from build123d import *

# Parameters (mm, degrees)
SKETCH7_R           = 2.5
BOSS_EXTRUDE3_DEPTH = 37
SKETCH8_W           = 15.4
SKETCH8_H           = 31
SKETCH8_W_2         = 8.010366446
SKETCH8_W_3         = 36.155804789
CUT_EXTRUDE4_DEPTH  = 76.893008599


with BuildPart() as part:
    # Sketch7 → Boss-Extrude3 (new body)
    with BuildSketch(Plane(origin=(0, 0, 0), x_dir=(1, 0, 0), z_dir=(0, 1, 0))):
        with BuildLine():
            Line((13.729937465, 55.269451431), (59.029937465, 55.269451431))
            ThreePointArc((59.029937465, 55.269451431), (65.129937465, 49.169451431), (59.029937465, 43.069451431))
            Line((59.029937465, 43.069451431), (13.729937465, 43.069451431))
            ThreePointArc((13.729937465, 43.069451431), (7.629937465, 49.169451431), (13.729937465, 55.269451431))
        make_face()
        with Locations(Location((13.729937465, 49.169451431, 0), (0, 0, 270))):
            Circle(SKETCH7_R, mode=Mode.SUBTRACT)
        with Locations(Location((59.029937465, 49.169451431, 0), (0, 0, 270))):
            Circle(SKETCH7_R, mode=Mode.SUBTRACT)
    extrude(amount=BOSS_EXTRUDE3_DEPTH)

    # Sketch8 → Cut-Extrude4 (cut, through all)
    with BuildSketch(Plane(origin=(0, 0, -55.269451431), x_dir=(-1, 0, 0), z_dir=(0, 0, -1))):
        with Locations((-21.429937465, 18.5)):
            Rectangle(SKETCH8_W, SKETCH8_H)
        with Locations((-9.724754242, 18.5)):
            Rectangle(SKETCH8_W_2, SKETCH8_H)
        with Locations((-50.207839859, 18.5)):
            Rectangle(SKETCH8_W_3, SKETCH8_H)
    extrude(amount=-CUT_EXTRUDE4_DEPTH, mode=Mode.SUBTRACT)


solid = part.part
The listing builds one solid part. Answer for the finished solid, in the listing's coordinates (mm). A direction names the side the tool comes from. Round coordinates to 2 decimals unless told otherwise and drop trailing zeros. Loops run counter-clockwise (first coordinate to the right, second up) from the corner with the lowest first, then second, coordinate; pieces in that order, holes last. Notation, with made-up numbers: M 86.25,52.5 L 115.25,52.5 A27 cw 115.25,68.5 Z; hole C -25,-30 d10. An arc over 180 degrees is marked long. Return JSON: item names as keys, results as strings.
Q1. Find section A-A, the plane x = 37. Determine the outline of the cut face in (y, z).
Results list:
{"outline": "M 0,-55.27 L 3,-55.27 L 3,-43.07 L 0,-43.07 Z; M 34,-55.27 L 37,-55.27 L 37,-43.07 L 34,-43.07 Z"}
Q2. The mould has two halves that part along Y. Classify faces 1 (the face through (37, 37, -49)), 2 (the face through (7.63, 1.48, -49.04)), 3 (the face through (29.13, 18, -49)), 4 (the face through (49, 34, -49)): released by +Y, released by -Y, zero draft, split by the parting line, or undercut.
Results list:
{"face 1": "released by +Y", "face 2": "zero draft", "face 3": "undercut", "face 4": "undercut"}
Q3. Find section C-C, the plane z = -52.5. Determine the outline of the cut face in (x, y), plus the area to 3 significant figures.
Results list:
{"outline": "M 8.62,0 L 64.14,0 L 64.14,3 L 32.13,3 L 32.13,34 L 64.14,34 L 64.14,37 L 8.62,37 L 8.62,34 L 29.13,34 L 29.13,3 L 8.62,3 Z", "area": "426 mm2"}
Q4. Each of these flat-tipped pins is pushed along its axis until it touches: pin 1 Ø5 at (y, z) = (29.5, -52) entering from +X; pin 2 Ø1 at (y, z) = (30, -50) entering from -X. Where does it stop, or does it pass through?
Results list:
{"pin 1": "stops at x = 32.13", "pin 2": "stops at x = 29.13"}
Q5. Which of the six approach directions +Z, -Z, +X, -X, +Y, -Y give full straight-line access (tool end or side, diameter ignored) to faces 5 (the face through (32.13, 18, -49)), 6 (the face through (18, 34, -49)), 7 (the face through (31, 20, -55.269))?
Results list:
{"face 5": "+Z, -Z, +X", "face 6": "+Z, -Z, -X", "face 7": "-Z, +X, -X, +Y, -Y"}
Q6. Find the intervals of material crossed by line 1 along Y through (x, z) = (50.5, -47.25); line 2 along X through (y, z) = (15, -45.25); line 3 along X through (y, z) = (2, -53.75), in increasing order. Write a range as from..to.
Results list:
{"line 1": "y = 0..3, 34..37", "line 2": "x = 29.13..32.13", "line 3": "x = 9.7..63.06"}
Q7. Find section D-D, the plane x = 58. Determine the outline of the cut face in (y, z), plus the area to 3 significant figures.
Results list:
{"outline": "M 0,-55.27 L 3,-55.27 L 3,-51.45 L 0,-51.45 Z; M 0,-46.89 L 3,-46.89 L 3,-43.07 L 0,-43.07 Z; M 34,-55.27 L 37,-55.27 L 37,-51.45 L 34,-51.45 Z; M 34,-46.89 L 37,-46.89 L 37,-43.07 L 34,-43.07 Z", "area": "45.9 mm2"}
Q8. Find section B-B, the plane z = -48.75. Determine the outline of the cut face in (x, y), plus the area to 3 significant figures.
Results list:
{"outline": "M 7.64,0 L 11.27,0 L 11.27,3 L 7.64,3 Z; M 7.64,34 L 11.27,34 L 11.27,37 L 7.64,37 Z; M 16.19,0 L 56.57,0 L 56.57,3 L 32.13,3 L 32.13,34 L 56.57,34 L 56.57,37 L 16.19,37 L 16.19,34 L 29.13,34 L 29.13,3 L 16.19,3 Z; M 61.49,0 L 65.12,0 L 65.12,3 L 61.49,3 Z; M 61.49,34 L 65.12,34 L 65.12,37 L 61.49,37 Z", "area": "379 mm2"}
